For this review, take the finished solid that the model builds, in its own axes (mm). Face numbers are marked on the shaded views. A direction names the side the tool comes from. Give positions to 0.01 mm unless a question says otherwise; leave off trailing zeros. Loops run counter-clockwise (first coordinate to the right, second up) from the corner with the lowest first, then second, coordinate; pieces in that order, holes last. Notation, with made-up numbers: M -4,-11.5 L 39,-11.5 A11 ccw 39,-7.5 Z; hole C 5,10 d7. An arc over 180 degrees is marked long. Use CSV: the item, a comma, the result in double quotes. Start each with the question number.
1. To check wall thickness, follow line 1 (X direction, y = 33.65, z = 10.5); line 2 (Y direction, x = 0, z = -6.15); line 3 (X direction, y = 0.5, z = 0). State the ranges of each line that lie inside material, in increasing order. Write a range as [from, to].
2. The part is to be moulded in two halves that separate along Z. For the marked faces 1, 2 and 3, say which applies: pulls with the +Z half, pulls with the -Z half, needs draft (parallel to the pull), parting line crosses it, or undercut.
3. Take a section at D-D, the plane z = -13. Write out the cut boundary in (x, y), and give its area (3 significant figures).
4. Take a section at A-A, the plane y = -11.1. Write out the cut boundary in (x, z).
5. Take a section at B-B, the plane z = -21. Write out the cut boundary in (x, y), and give its area (3 significant figures).
6. Tool access review of the marked faces 4, 5, 6 and 7: name each direction out of +Z, -Z, +X, -X, +Y, -Y from which nothing blocks a thin tool from reaching the whole face with its end or side.
7. Insertion check: P1, Ø5, axis at y = 14, z = 5, coming from the -X side; P2, Ø8, axis at y = -12.5, z = -1, coming from the +X side; P3, Ø1.5, axis at x = -7.5, z = -19.5, coming from the -Y side; P4, Ø17.5, axis at x = -3, z = -2.5, coming from the -Y side. Each pin has a flat end and moves straight along its axis. Give the tip position at first contact, or say it passes through.
8. Take a section at C-C, the plane y = 27. Write out the cut boundary in (x, z), and give its area (3 significant figures).
from build123d import *
from build123d.topology import SkipClean

# Parameters (mm, degrees)
EXTRUDE_START       = 21
EXTRUDE_1_DEPTH     = 21
SKETCH_5_R          = 2.5
CUT_EXTRUDE_1_DEPTH = 64.460932864
CHAMFER_1_SIZE      = 0.5
FILLET_1_R          = 2
SKETCH_9_R          = 1.5
CUT_EXTRUDE_2_DEPTH = 62.947473135
CUT_EXTRUDE_4_DEPTH = 21


with BuildPart() as part:
    # 草图2 → 旋转1 (revolve)
    with BuildSketch(Plane.XY, mode=Mode.PRIVATE) as revolve_1_sk:
        Polygon((0, 0), (0, 49.7), (10, 49.7), (10, 34.7), (25, 34.7), (25, 31.7), (9, 31.7), (9, 22.7), (8.5, 22.7), (8.5, 18.2), (8, 18.2), (8, 7.5), (8.5, 7.5), (8.5, 2.5), (8, 2.5), (7.2, 2.5), (7.2, 1.5), (8, 1.5), (8, 0), align=None)
    revolve(revolve_1_sk.sketch.rotate(Axis((0, 0, 0), (0, 1, 0)), 90), axis=Axis((0, 0, 0), (0, 1, 0)))

    # 草图3 → 凸台-拉伸1 (add)
    with BuildSketch(Plane.XZ.offset(EXTRUDE_START)):
        with BuildLine():
            Line((-7.039886363, 3.8), (-3.249615362, 3.8))
            ThreePointArc((-3.249615362, 3.8), (0, -5), (3.249615362, 3.8))
            Line((3.249615362, 3.8), (7.039886363, 3.8))
            ThreePointArc((7.039886363, 3.8), (0, -8), (-7.039886363, 3.8))
        make_face()
    extrude(amount=-EXTRUDE_1_DEPTH)

    # 草图5 → 切除-拉伸1 (cut, through all)
    with BuildSketch(Plane.XZ.offset(-31.7)):
        with BuildLine():
            ThreePointArc((-4.80408962, -24.534072693), (-9.959292144, -5.75), (-23.649175021, 8.106572693))
            ThreePointArc((-23.649175021, 8.106572693), (-21.650635095, -12.5), (-4.80408962, -24.534072693))
        make_face()
        with BuildLine():
            ThreePointArc((25, 0), (24.659981504, 4.109174155), (23.649175021, 8.106572693))
            ThreePointArc((23.649175021, 8.106572693), (9.959292144, -5.75), (4.80408962, -24.534072693))
            ThreePointArc((4.80408962, -24.534072693), (19.301583361, -15.888639959), (25, 0))
        make_face()
        with BuildLine():
            ThreePointArc((18.8450854, 16.4275), (0, 25), (-18.8450854, 16.4275))
            ThreePointArc((-18.8450854, 16.4275), (0, 11.5), (18.8450854, 16.4275))
        make_face()
        with Locations(Location((0, -21, 0), (0, 0, 270))):
            Circle(SKETCH_5_R)
        with Locations(Location((18.186533479, 10.5, 0), (0, 0, 270))):
            Circle(SKETCH_5_R)
        with Locations(Location((-18.186533479, 10.5, 0), (0, 0, 270))):
            Circle(SKETCH_5_R)
    extrude(amount=-CUT_EXTRUDE_1_DEPTH, mode=Mode.SUBTRACT)

    # 倒角1
    chamfer_1_edges = [part.edges().sort_by_distance(p)[0] for p in [
        (0, 2.5, 8.5),
        (0, 18.2, 8),
        (0, 31.7, 9),
        (0, 49.7, 10),
    ]]
    chamfer(chamfer_1_edges, length=CHAMFER_1_SIZE - 0.0001)  # a hair under: the kernel refuses the full size

    # 圆角1
    fillet_1_edges = [part.edges().sort_by_distance(p)[0] for p in [
        (-18.8450854, 33.2, 16.4275),
        (18.8450854, 33.2, 16.4275),
        (23.649175021, 33.2, 8.106572693),
        (4.80408962, 33.2, -24.534072693),
        (-4.80408962, 33.2, -24.534072693),
        (-23.649175021, 33.2, 8.106572693),
    ]]
    fillet(fillet_1_edges, radius=FILLET_1_R)

    # 草图8 → 切除-旋转1 (revolve, cut)
    with BuildSketch(Plane.XY, mode=Mode.PRIVATE) as cut_revolve_1_sk:
        Polygon((8, 34.7), (5, 34.7), (5, 0), (0, 0), (0, 49.7), (8, 49.7), align=None)
    revolve(cut_revolve_1_sk.sketch.rotate(Axis((0, 49.7, 0), (0, -1, 0)), 270), axis=Axis((0, 49.7, 0), (0, -1, 0)), mode=Mode.SUBTRACT)

    # 草图9 → 切除-拉伸2 (cut, through all)
    with SkipClean():  # the faces are left unmerged after this step: merging them gives an invalid solid
        with BuildSketch(Plane.XY.offset(3.8)):
            with Locations((0, -11.1)):
                Circle(SKETCH_9_R)
        extrude(amount=-CUT_EXTRUDE_2_DEPTH, mode=Mode.SUBTRACT)

    # 草图11 → 切除-拉伸4 (cut)
    with SkipClean():  # the faces are left unmerged after this step: merging them gives an invalid solid
        with BuildSketch(Plane.XZ.offset(21)):
            with BuildLine():
                Line((-7.039886363, 3.8), (-7.039886363, -3.8))
                ThreePointArc((-7.039886363, -3.8), (-8, 0), (-7.039886363, 3.8))
            make_face()
            with BuildLine():
                Line((7.039886363, 3.8), (7.039886363, -3.8))
                ThreePointArc((7.039886363, -3.8), (8, 0), (7.039886363, 3.8))
            make_face()
        extrude(amount=-CUT_EXTRUDE_4_DEPTH, mode=Mode.SUBTRACT)


solid = part.part
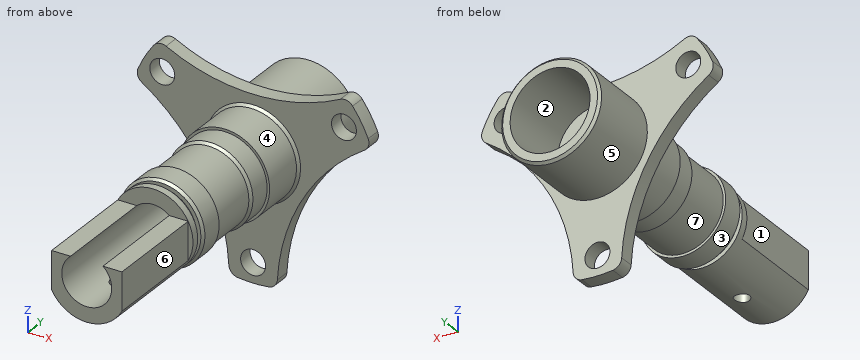
Result set:
1,line 1,"[-22.69, -20.69], [-15.69, 15.69], [20.69, 22.69]"
1,line 2,"[-21, -12.6], [-9.6, 34.7]"
1,line 3,"[-8, -5], [5, 8]"
2,face 1,"needs draft"
2,face 2,"undercut"
2,face 3,"parting line crosses it"
3,outline,"M -6.72,31.7 L 6.72,31.7 L 6.72,34.7 L -6.72,34.7 Z"
3,area,"40.3 mm2"
4,outline,"M -7.04,-3.8 A8 ccw -1.5,-7.86 L -1.5,-4.77 A5 cw -3.25,3.8 L -7.04,3.8 Z; M 1.5,-7.86 A8 ccw 7.04,-3.8 L 7.04,3.8 L 3.25,3.8 A5 cw 1.5,-4.77 Z"
5,outline,"M -5.01,31.7 L -2.5,31.7 L -2.5,34.7 L -5.01,34.7 Z; M 2.5,31.7 L 5.01,31.7 L 5.01,34.7 L 2.5,34.7 Z"
5,area,"15.1 mm2"
6,face 4,"-Y"
6,face 5,"+Y"
6,face 6,"+Z, -Z, +X, -Y"
6,face 7,"none"
7,P1,"x = -7.6"
7,P2,"x = 7.04"
7,P3,"through"
7,P4,"y = -21"
8,outline,"C 0,0 d18; hole C 0,0 d10"
8,area,"176 mm2"
